Geometry check sheet. Reference: drawing and pictorial views, mm from the part's lowest x, y, z. A direction names the side the tool comes from. Round coordinates to 2 decimals unless told otherwise and drop trailing zeros. Loops run counter-clockwise (first coordinate to the right, second up) from the corner with the lowest first, then second, coordinate; pieces in that order, holes last. Notation, with made-up numbers: (-18, -35.5) -> (17, -35.5) arc R26 cw to (17, -21.5) -> close; hole circle Ø5 at (53, 75). An arc over 180 degrees is marked (long way). Use one line per item in the form item = value. Start each with the question number.
(1) Sectioned sample at A-A (y = 16.5). Record the cut outline in (x, z).
(2) Sectioned sample at C-C (y = 7). Record the cut outline in (x, z), and give its area (3 significant figures).
(3) Set-up check for the marked faces 1, 2 and 3: record each of +Z, -Z, +X, -X, +Y, -Y from which the full face is reachable in a straight line by a thin tool's end or side.
(4) Draft check along X on the marked faces 4, 5 and 6. Enter one of: released by +X, released by -X, zero draft, split by the parting line, or undercut.
(5) Sectioned sample at D-D (x = 29.5). Record the cut outline in (y, z).
(6) Go/stop test with flat-tipped pins: pin 1 (1.4 mm diameter, centred on y = 10, z = 12, fed in from -X); pin 2 (2 mm diameter, centred on x = 33.5, z = 6.5, fed in from +Y); pin 3 (1 mm diameter, centred on x = 17, z = 7.5, fed in from +Y). Record where each tip stops, or that it passes through.
(7) Material ranges on probe 1 along X at (y, z) = (11, 6.75); probe 2 along X at (y, z) = (16.75, 5.75); probe 3 along X at (y, z) = (2.25, 3), recorded low to high. Write a range as [from, to].
(8) Sectioned sample at B-B (z = 6.5). Record the cut outline in (x, y).
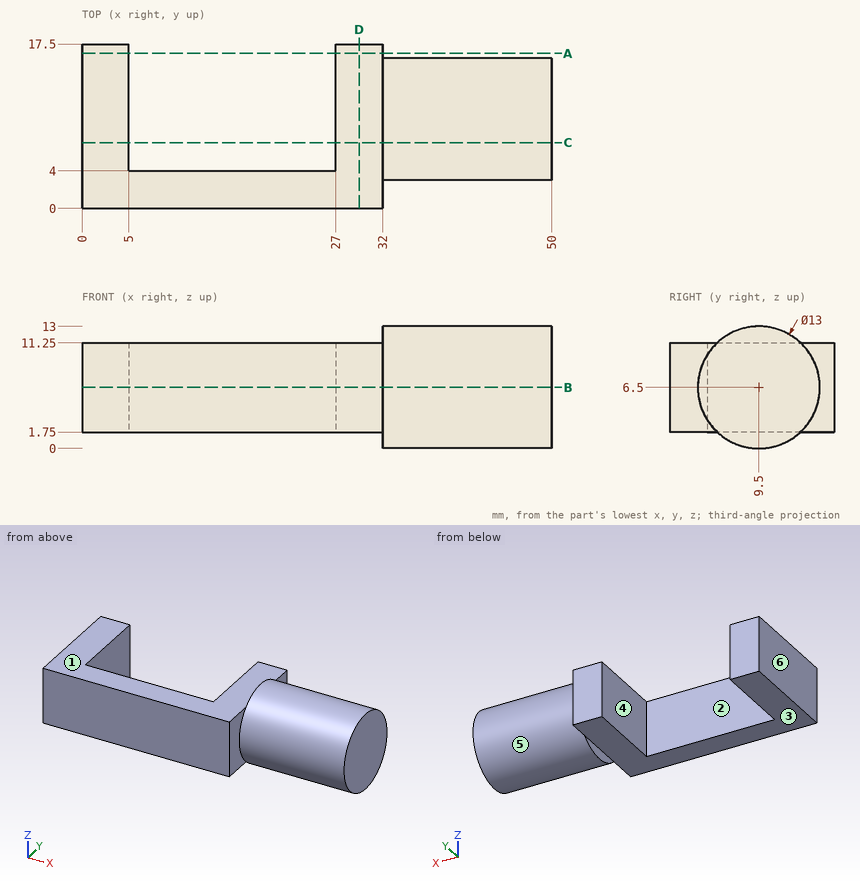
Checks:
q1.outline = (0, 1.75) -> (5, 1.75) -> (5, 11.25) -> (0, 11.25) -> close; (27, 1.75) -> (32, 1.75) -> (32, 11.25) -> (27, 11.25) -> close
q2.outline = (0, 1.75) -> (5, 1.75) -> (5, 11.25) -> (0, 11.25) -> close; (27, 1.75) -> (32, 1.75) -> (32, 0.5) -> (50, 0.5) -> (50, 12.5) -> (32, 12.5) -> (32, 11.25) -> (27, 11.25) -> close
q2.area = 311 mm2
q3.face_1 = +Z, -X, +Y, -Y
q3.face_2 = +Z, -Z, +Y
q3.face_3 = -Z, -X, +Y, -Y
q4.face_4 = undercut
q4.face_5 = zero draft
q4.face_6 = released by -X
q5.outline = (0, 1.75) -> (17.5, 1.75) -> (17.5, 11.25) -> (0, 11.25) -> close
q6.pin_1 = 32
q6.pin_2 = 16
q6.pin_3 = 4
q7.probe_1 = [0, 5], [27, 50]
q7.probe_2 = [0, 5], [27, 32]
q7.probe_3 = [0, 32]
q8.outline = (0, 0) -> (32, 0) -> (32, 3) -> (50, 3) -> (50, 16) -> (32, 16) -> (32, 17.5) -> (27, 17.5) -> (27, 4) -> (5, 4) -> (5, 17.5) -> (0, 17.5) -> close
